Here's how the part is built. I have some questions about the finished solid (model axes, mm). A direction names the side the tool comes from. Coordinates: 2 decimals unless noted, no trailing zeros. Write each loop counter-clockwise with the first axis right and the second up, starting at its lowest first coordinate (ties: lowest second). Pieces come first, ordered by that corner, then holes.
(1) For pin 1 Ø6 at (y, z) = (-0.5, 13) entering from +X; pin 2 Ø4 at (y, z) = (-0.5, 13.5) entering from -X; pin 3 Ø1 at (y, z) = (-3, 22.5) entering from -X, each with a flat end and sliding along its axis, tell me the tip position at first contact or that it passes through.
(2) Imagine slicing it at A-A, the plane z = 31.5. List the corners of the cut face in (x, y) for me.
(3) Imagine slicing it at B-B, the plane z = 8.5. List the corners of the cut face in (x, y) for me, plus the area to 3 significant figures.
(4) Which directions (+Z, -Z, +X, -X, +Y, -Y) give clear straight access to the entire face, cutting with the end or side of a thin tool? Please do faces 4 (the cylindrical face through (-11.92, -9.14, 3.47)), 5 (the flat face through (4, -7, 26)), 6 (the cylindrical face through (8.82, 2.78, 22.45)).
(5) Please list where these lines run through material, in increasing order: probe 1 along Y at (x, z) = (0, 13); probe 2 along Z at (x, y) = (-3, -8.5); probe 3 along Z at (x, y) = (8.5, -5).
(6) Thinking about a two-plate mould opening in Y: for faces 1 (the cylindrical face through (-3.3, 3.03, 18.73)), 2 (the cylindrical face through (-9.236, 0.406, 29.479)), 3 (the flat face through (0, -6, 0)), which applies, released by +Y, released by -Y, zero draft, split by the parting line, or undercut?
```python
from build123d import *

# Parameters (mm, degrees)
F0_R      = 15.020122
F1_DEPTH  = 7
F2_R      = 11.015093
F3_DEPTH  = 12
F4_R      = 9.249668
F5_DEPTH  = 7
F6_R      = 7.745011
F7_DEPTH  = 2
F8_R      = 9.244849
F9_DEPTH  = 3
F10_R     = 7.744613
F11_DEPTH = 2
F12_R     = 9.247202
F13_DEPTH = 5
F14_SIZE  = 1.5
F15_R     = 1.5
F16_R     = 4.480588
F17_DEPTH = 50


with BuildPart() as f1:
    # F0 (on Top) → F1 (new body)
    with BuildSketch(Plane.XY):
        Circle(F0_R)
    extrude(amount=F1_DEPTH)

    # F2 (on face) → F3 (join)
    with BuildSketch(Plane.XY.offset(7)):
        Circle(F2_R)
    extrude(amount=F3_DEPTH)

    # F4 (on face) → F5 (join)
    with BuildSketch(Plane.XY.offset(19)):
        Circle(F4_R)
    extrude(amount=F5_DEPTH)

    # F6 (on face) → F7 (join)
    with BuildSketch(Plane.XY.offset(26)):
        Circle(F6_R)
    extrude(amount=F7_DEPTH)

    # F8 (on face) → F9 (join)
    with BuildSketch(Plane.XY.offset(28)):
        Circle(F8_R)
    extrude(amount=F9_DEPTH)

    # F10 (on face) → F11 (join)
    with BuildSketch(Plane.XY.offset(31)):
        Circle(F10_R)
    extrude(amount=F11_DEPTH)

    # F12 (on face) → F13 (join)
    with BuildSketch(Plane.XY.offset(33)):
        Circle(F12_R)
    extrude(amount=F13_DEPTH)

    # F14
    f14_edges = [f1.edges().sort_by_distance(p)[0] for p in [
        (-9.247202, 0, 38),
    ]]
    chamfer(f14_edges, length=F14_SIZE)

    # F15
    f15_edges = [f1.edges().sort_by_distance(p)[0] for p in [
        (-15.020122, 0, 7),
        (-15.020122, 0, 0),
    ]]
    fillet(f15_edges, radius=F15_R)

    # F16 (on Top) → F17 (cut)
    with BuildSketch(Plane.XY):
        Circle(F16_R)
    extrude(amount=F17_DEPTH, mode=Mode.SUBTRACT)


solid = f1.part
```
Recorded:
1. pin 1: stops at x = 11.02
1. pin 2: stops at x = -11.02
1. pin 3: stops at x = -8.91
2. outline: circle Ø15.49 at (0, 0); hole circle Ø8.96 at (0, 0)
3. outline: circle Ø22.03 at (0, 0); hole circle Ø8.96 at (0, 0)
3. area: 318 mm2
4. face 4: +Z, -Z
4. face 5: none
4. face 6: +Z
5. probe 1: y = -11.02 to -4.48, 4.48 to 11.02
5. probe 2: z = 0 to 26, 28 to 31, 33 to 36.73
5. probe 3: z = 0 to 19
6. face 1: undercut
6. face 2: split by the parting line
6. face 3: zero draft
